Source: CAD feature listing. Evaluate the final solid. Frame: model axes, mm. A direction names the side the tool comes from. Give positions to 0.01 mm unless a question says otherwise; leave off trailing zeros. Write each loop counter-clockwise with the first axis right and the second up, starting at its lowest first coordinate (ties: lowest second). Pieces come first, ordered by that corner, then holes. Notation, with made-up numbers: (62.25, -0.5) -> (112.25, -0.5) arc R31 ccw to (112.25, 23.5) -> close; hole circle Ø8 at (54.25, 47.5). An arc over 180 degrees is marked (long way). Use one line per item in the form item = value. Start each with the question number.
(1) Cut plane B-B, the plane x = 0. Output: boundary loops of the cut face in (y, z), and give its area (3 significant figures).
(2) Cut plane D-D, the plane z = -23. Output: boundary loops of the cut face in (x, y).
(3) Material intervals for line 1 along X through (y, z) = (10.25, 0); line 2 along Y through (x, z) = (9.5, 10.5); line 3 along X through (y, z) = (3, 20.5), sorted ascending. Write a range as from..to.
(4) Draft query along Z for faces 5 (the face through (-11.49, 8.381, 27.712)), 6 (the face through (29, 7, -9)), 7 (the face through (16.7, 7, 16.3)). Return one class per face: pulls with the +Z half, pulls with the -Z half, needs draft (parallel to the pull), parting line crosses it, or undercut.
(5) Cut plane C-C, the plane z = 6. Output: boundary loops of the cut face in (x, y), and give its area (3 significant figures).
(6) First-contact query: P1, Ø2.5, axis at x = 44.5, y = 0, coming from the -Z side; P2, Ø10, axis at y = 6, z = 12, coming from the -X side; P3, Ø1.4, axis at x = 29, z = 5.5, coming from the -Y side. Flat tips, straight axial feed; report the tip coordinate or a pass-through.
(7) Set-up query: faces 1 (the face through (-37, 3, 12.5)), 2 (the face through (-29, 2, -10)), 3 (the face through (-18, 11, 15)), 4 (the face through (37, 3, -12.5)). Return all of +Z, -Z, +X, -X, +Y, -Y with unobstructed straight access to the full face (end or side cutting, diameter ignored); none if empty.
(8) Cut plane A-A, the plane z = -10. Output: boundary loops of the cut face in (x, y), and give its area (3 significant figures).
from build123d import *

# Parameters (mm, degrees)
SKETCH1_R                = 30
BOSS_EXTRUDE1_DEPTH      = 17
SKETCH2_R                = 29
CUT_EXTRUDE1_DEPTH       = 15
SKETCH3_R                = 3
BOSS_EXTRUDE5_DEPTH      = 5
SKETCH4_R                = 1.5
BOSS_EXTRUDE6_DEPTH      = 4
BOSS_EXTRUDE7_REACH      = 71.203
BOSS_EXTRUDE7_END_RADIUS = 30
SKETCH6_W                = 25
SKETCH6_H                = 5
SKETCH9_W                = 25
SKETCH9_H                = 5
SKETCH10_W               = 3
SKETCH10_H               = 22
CUT_EXTRUDE2_DEPTH       = 10
CIRPATTERN1_COUNT        = 2


with BuildPart() as part:
    # Sketch1 → Boss-Extrude1 (new body)
    with BuildSketch(Plane(origin=(0, 0, 0), x_dir=(1, 0, 0), z_dir=(0, 1, 0))):
        with Locations(Location((0, 0, 0), (0, 0, 270))):
            Circle(SKETCH1_R)
    extrude(amount=BOSS_EXTRUDE1_DEPTH)

    # Sketch2 → Cut-Extrude1 (cut)
    with BuildSketch(Plane(origin=(0, 17, 0), x_dir=(1, 0, 0), z_dir=(0, 1, 0))):
        with Locations(Location((0, 0, 0), (0, 0, 270))):
            Circle(SKETCH2_R)
    extrude(amount=-CUT_EXTRUDE1_DEPTH, mode=Mode.SUBTRACT)

    # Sketch3 → Boss-Extrude5 (add)
    with BuildSketch(Plane(origin=(0, 2, 0), x_dir=(1, 0, 0), z_dir=(0, 1, 0))):
        with Locations(Location((-18, 15, 0), (0, 0, 270))):
            Circle(SKETCH3_R)
        with Locations(Location((-18, -15, 0), (0, 0, 270))):
            Circle(SKETCH3_R)
        with Locations(Location((18, -15, 0), (0, 0, 270))):
            Circle(SKETCH3_R)
        with Locations(Location((18, 15, 0), (0, 0, 270))):
            Circle(SKETCH3_R)
    extrude(amount=BOSS_EXTRUDE5_DEPTH)

    # Sketch4 → Boss-Extrude6 (add)
    with BuildSketch(Plane(origin=(0, 7, 0), x_dir=(1, 0, 0), z_dir=(0, 1, 0))):
        with Locations(Location((-18, 15, 0), (0, 0, 270))):
            Circle(SKETCH4_R)
        with Locations(Location((-18, -15, 0), (0, 0, 270))):
            Circle(SKETCH4_R)
        with Locations(Location((18, 15, 0), (0, 0, 270))):
            Circle(SKETCH4_R)
        with Locations(Location((18, -15, 0), (0, 0, 270))):
            Circle(SKETCH4_R)
    extrude(amount=BOSS_EXTRUDE6_DEPTH)

    # Boss-Extrude7: up to this cylinder (the profile starts outside it)
    boss_extrude7_end = Plane(origin=(0, 4.5, 0), z_dir=(0, -1, 0)) * Cylinder(BOSS_EXTRUDE7_END_RADIUS, 203.406, mode=Mode.PRIVATE)
    # Sketch6 → Boss-Extrude7 (add, up to the surface)
    with BuildSketch(Plane.ZY.offset(30), mode=Mode.PRIVATE) as boss_extrude7_sk1:
        with Locations((0, 4.5)):
            Rectangle(SKETCH6_W, SKETCH6_H)
    boss_extrude7_tool1 = extrude(boss_extrude7_sk1.sketch, amount=-BOSS_EXTRUDE7_REACH, mode=Mode.PRIVATE) - boss_extrude7_end
    boss_extrude7 = boss_extrude7_tool1.solids().sort_by_distance((-30, 4.5, 0))[0] + boss_extrude7_tool1.solids().sort_by_distance((-30, 4.5, 0))[1]
    add(boss_extrude7)

    # Sweep1: sweep along a path in Sketch7
    with BuildLine(Plane.XY) as sweep1_path:
        ThreePointArc((-30, 4.5), (-38.878296183, 2.772912041), (-46.461716328, -2.156460621))
    # Sketch9 → Sweep1 (sweep)
    with BuildSketch(Plane.ZY.offset(30)):
        with Locations((0, 4.5)):
            Rectangle(SKETCH9_W, SKETCH9_H)
    sweep1 = sweep(path=sweep1_path.line)

    # Sketch10 → Cut-Extrude2 (cut)
    with BuildSketch(Plane(origin=(-23.106823791, 23.900351253, 0), x_dir=(0.7189410106609229, 0.6950710921839945, 0), z_dir=(-0.6950710921839945, 0.7189410106609229, 0))):
        with Locations((-31.902126733, 0)):
            Rectangle(SKETCH10_W, SKETCH10_H)
    cut_extrude2 = extrude(amount=-CUT_EXTRUDE2_DEPTH, mode=Mode.SUBTRACT)

    # CirPattern1: Boss-Extrude7, Sweep1, Cut-Extrude2 ×2 about axis
    cirpattern1_axis = Axis((0, 0, 0), (0, 1, 0))
    add([boss_extrude7.rotate(cirpattern1_axis, i * 360 / CIRPATTERN1_COUNT) for i in range(1, CIRPATTERN1_COUNT)])
    add([sweep1.rotate(cirpattern1_axis, i * 360 / CIRPATTERN1_COUNT) for i in range(1, CIRPATTERN1_COUNT)])
    add([cut_extrude2.rotate(cirpattern1_axis, i * 360 / CIRPATTERN1_COUNT) for i in range(1, CIRPATTERN1_COUNT)], mode=Mode.SUBTRACT)


solid = part.part
Geometry says:
q1.outline = (0, -30) -> (17, -30) -> (17, -29) -> (2, -29) -> (2, 29) -> (17, 29) -> (17, 30) -> (0, 30) -> close
q1.area = 150 mm^2
q2.outline = (-19.26, 0) -> (19.26, 0) -> (19.26, 17) -> (17.66, 17) -> (17.66, 2) -> (-17.66, 2) -> (-17.66, 17) -> (-19.26, 17) -> close
q3.line_1 = -30..-29, 29..30
q3.line_2 = 0..2
q3.line_3 = -21.9..-20.51, 20.51..21.9
q4.face_5 = parting line crosses it
q4.face_6 = needs draft
q4.face_7 = undercut
q5.outline = (-48.2, -0.36) -> (-44.72, -3.95) arc R21.18 cw to (-43.61, -2.95) -> (-47.09, 0.65) arc R26.18 ccw to start; (-44.69, 2.49) -> (-41.15, -1.17) arc R21.18 cw to (-30, 2) -> (-29.39, 2) -> (-29.39, 0) -> (29.39, 0) -> (29.39, 2) -> (30, 2) arc R21.18 cw to (41.15, -1.17) -> (44.69, 2.49) arc R26.18 ccw to (30, 7) -> (29.39, 7) -> (29.39, 17) -> (28.37, 17) -> (28.37, 2) -> (-28.37, 2) -> (-28.37, 17) -> (-29.39, 17) -> (-29.39, 7) -> (-30, 7) arc R26.18 ccw to start; (43.61, -2.95) arc R21.18 cw to (44.72, -3.95) -> (48.2, -0.36) arc R26.18 ccw to (47.09, 0.65) -> close
q5.area = 306 mm^2
q6.P1 = -12.5
q6.P2 = -46.68
q6.P3 = 0
q7.face_1 = +Z, -X, +Y, -Y
q7.face_2 = -Z, -Y
q7.face_3 = +Y
q7.face_4 = -Z, +X, +Y, -Y
q8.outline = (-48.2, -0.36) -> (-44.72, -3.95) arc R21.18 cw to (-43.61, -2.95) -> (-47.09, 0.65) arc R26.18 ccw to start; (-44.69, 2.49) -> (-41.15, -1.17) arc R21.18 cw to (-30, 2) -> (-28.28, 2) -> (-28.28, 0) -> (28.28, 0) -> (28.28, 2) -> (30, 2) arc R21.18 cw to (41.15, -1.17) -> (44.69, 2.49) arc R26.18 ccw to (30, 7) -> (28.28, 7) -> (28.28, 17) -> (27.22, 17) -> (27.22, 2) -> (-27.22, 2) -> (-27.22, 17) -> (-28.28, 17) -> (-28.28, 7) -> (-30, 7) arc R26.18 ccw to start; (43.61, -2.95) arc R21.18 cw to (44.72, -3.95) -> (48.2, -0.36) arc R26.18 ccw to (47.09, 0.65) -> close
q8.area = 314 mm^2
